Can you work these out from the model? Positions are in its coordinate system, mm. Face numbers are marked on the shaded views. A direction names the side the tool comes from. Give positions to 0.01 mm unless a question says otherwise; leave off trailing zeros. Order: outer loops, then holes, each group sorted by start corner. A loop starts at its lowest first (then second) coordinate and runs counter-clockwise, first axis right, second up. Notation, with made-up numbers: M 82,20.5 L 136,20.5 A22 cw 136,30.5 Z; hole C 16.25,69.25 d8. An arc over 180 degrees is marked long. Answer as a JSON object with one key per item and string values.
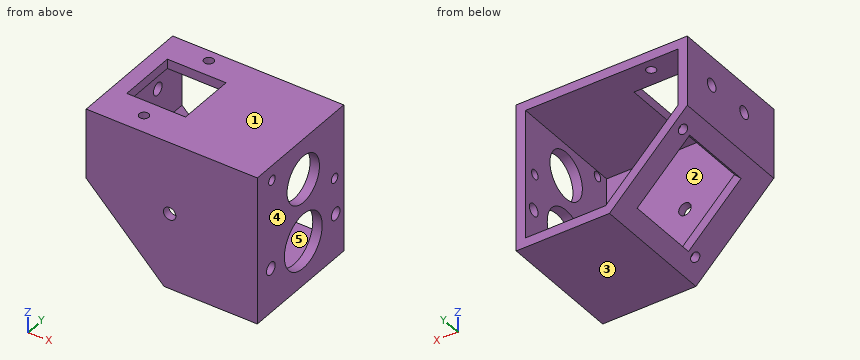
Autodesk Inventor part; units mm, degrees
ref_plane "YZ Plane" through (0, 0, 0) normal (1, 0, 0) x (0, 1, 0)
ref_plane "XZ Plane" through (0, 0, 0) normal (0, 1, 0) x (-1, 0, 0)
ref_plane "XY Plane" through (0, 0, 0) normal (0, 0, 1) x (1, 0, 0)
sketch "Sketch1" plane through (0, 0, 0) normal (0, 1, 0) x (-1, 0, 0)
  line L0 (0, -4) -> (15, -4) construction
  line L1 (15, -4) -> (15, -12) construction
  line L2 (15, -12) -> (-4.6836, -12) construction
  line L3 (0, 0) -> (19.4569, 0)
  line L4 (19.4569, 0) -> (19.4569, -7.2603)
  line L5 (10.2172, -16.5) -> (0, -16.5)
  line L6 (0, -16.5) -> (0, 0)
  line L7 (-1.2, 1.2) -> (20.6569, 1.2)
  line L8 (20.6569, 1.2) -> (20.6569, -7.7574)
  line L9 (10.7142, -17.7) -> (-1.2, -17.7)
  line L10 (-1.2, -17.7) -> (-1.2, 1.2)
  line L11 (10.2172, -16.5) -> (19.4569, -7.2603)
  line L12 (20.6569, -7.7574) -> (10.7142, -17.7)
  line L13 (15, -12) -> (15.7071, -12.7071) construction
  line L14 (17.4749, -6.4749) -> (12.5251, -1.5251) construction
  line L15 (12.5251, -1.5251) -> (13.2676, -0.7827) construction
  line L16 (17.4749, -6.4749) -> (18.2173, -5.7324) construction
  line L17 (18.2173, -5.7324) -> (13.2676, -0.7827) construction
  line L18 (15, -12) -> (16.1863, -13.1863) construction
  point P0 (15, -8)
  dimension "d0" = 1.2
  dimension "d1" = 1.2
  dimension "d2" = 1.2
  dimension "d3" = 4
  dimension "d4" = 4.5
  dimension "d5" = 8
  dimension "d6" = 15
  dimension "d8" = 135
  dimension "d9" = 1.2
  dimension "d10" = 1.2
  dimension "d11" = 1
  dimension "d12" = 7
  dimension "d13" = 45
  dimension "d20" = 7
  dimension "d21" = 1.05
  dimension "d49" = 1.2395
  dimension "d68" = 4.4569
  dimension "d69" = 8
extrude "Extrusion1" add sketch "Sketch1" along normal mid plane 15
sketch "Sketch2" plane through (1.2, -7.5, -17.7) normal (1, 0, 0) x (0, 0, -1)
  circle A0 centre (-5.7, 7.5) radius 3.5
  circle A1 centre (-13.7, 7.5) radius 3
  circle A2 centre (-10.4, 13.3) radius 0.6
  circle A3 centre (-17, 1.7) radius 0.6
  line L0 (-10.4, 13.3) -> (-17, 1.7) construction
  line L1 (-16.7, 7.5) -> (-16.7, 7.5)
  circle A4 centre (-9.7, 1.5) radius 0.8
  line L2 (0, 0) -> (-18.9, 0)
  line L3 (-13.7, 7.5) -> (-5.7, 7.5) construction
  circle A5 centre (-5.7, 13.5) radius 0.8
  circle A6 centre (-5.7, 1.5) radius 0.8
  line L4 (-5.7, 1.5) -> (-5.7, 13.5) construction
  point P0 (-17.7, 7.5)
  point P1 (-5.7, 7.5)
  point P2 (-9.7, 7.5)
  dimension "d22" = 7
  dimension "d23" = 6
  dimension "d56" = 5.8
  dimension "d57" = 3.3
  dimension "d58" = 1.2
  dimension "d59" = 3
  dimension "d66" = 1.6
  dimension "d67" = 1.5
  dimension "d74" = 6
extrude "Extrusion2" cut sketch "Sketch2" against normal blind 3 contours A0 | A1 | A2 | A3 | A5 | A6
sketch "Sketch3" plane through (-20.6569, -7.5, 1.2) normal (-1, 0, 0) x (0, 0, 1)
  circle A0 centre (-3.7, 10.5) radius 0.8
  circle A1 centre (-5.2, 7.5) radius 0.8 construction
  circle A2 centre (-3.7, 4.5) radius 0.8
  line L0 (-11.5, 6.75) -> (-11.5, 8.25)
  line L1 (-9.9, 6.75) -> (-9.9, 8.25)
  arc A3 (-9.9, 8.25) -> (-11.5, 8.25) centre (-10.7, 8.25) ccw
  arc A4 (-11.5, 6.75) -> (-9.9, 6.75) centre (-10.7, 6.75) ccw
  line L2 (-3.7, 4.5) -> (-3.7, 10.5) construction
  point P0 (-1.2, 7.5)
  point P1 (-5.2, 7.5)
  point P2 (-10.7, 7.5)
  point P3 (-11.5, 7.5)
  point P4 (-3.7, 7.5)
  dimension "d28" = 1.6
  dimension "d32" = 5.5
  dimension "d52" = 1.5
  dimension "d53" = 0.8
  dimension "d64" = 6
  dimension "d65" = 1.5
extrude "Extrusion3" cut sketch "Sketch3" against normal blind 2 contours A0 | A2
sketch "Sketch4" plane through (-20.6569, -7.5, -7.7574) normal (-0.7071, 0, -0.7071) x (-0.7071, 0, 0.7071)
  line L0 (-11.75, 12.25) -> (-2.25, 12.25)
  line L1 (-2.25, 12.25) -> (-2.25, 2.75)
  line L2 (-2.25, 2.75) -> (-11.75, 2.75)
  line L3 (-11.75, 2.75) -> (-11.75, 12.25)
  circle A0 centre (-11.75, 13.5) radius 0.6
  circle A1 centre (-2.25, 13.5) radius 0.6
  circle A2 centre (-11.75, 1.5) radius 0.6
  circle A3 centre (-2.25, 1.5) radius 0.6
  point P0 (-9.1213, 7.5)
  point P1 (-7, 7.5)
  point P2 (-7, 7.5)
  point P3 (-7, 7.5)
  point P4 (-11.75, 7.5)
  point P5 (-7, 12.25)
  dimension "d35" = 9.5
  dimension "d36" = 6
  dimension "d37" = 6
  dimension "d38" = 1.2
extrude "Extrusion4" cut sketch "Sketch4" against normal blind 2 contours L0 L1 L2 L3 | A1 | A2
sketch "Sketch5" plane through (-20.6569, 7.5, 1.2) normal (0, 0, 1) x (1, 0, 0)
  line L0 (1.9069, -3.75) -> (9.4069, -3.75)
  line L1 (9.4069, -3.75) -> (9.4069, -11.25)
  line L2 (9.4069, -11.25) -> (1.9069, -11.25)
  line L3 (1.9069, -11.25) -> (1.9069, -3.75)
  circle A0 centre (5.6569, -1.5) radius 0.6
  circle A1 centre (5.6569, -13.5) radius 0.6
  arc A2 (13.6569, -12.7) -> (13.6569, -14.3) centre (13.6569, -13.5) ccw
  arc A3 (17.6569, -14.3) -> (17.6569, -12.7) centre (17.6569, -13.5) ccw
  line L4 (13.6569, -12.7) -> (17.6569, -12.7)
  line L5 (13.6569, -14.3) -> (17.6569, -14.3)
  point P0 (20.6569, -7.5)
  point P1 (5.6569, -7.5)
  point P2 (5.6569, -7.5)
  point P3 (5.6569, -7.5)
  point P4 (9.4069, -7.5)
  point P5 (5.6569, -3.75)
  point P6 (15.6569, -12.7)
  dimension "d41" = 7.5
  dimension "d42" = 6
  dimension "d43" = 6
  dimension "d44" = 1.2
  dimension "d70" = 1.6
  dimension "d71" = 6
  dimension "d72" = 10
  dimension "d73" = 4
extrude "Extrusion5" cut sketch "Sketch5" against normal blind 2 contours L0 L1 L2 L3 | A0 | A1
sketch "Sketch6" plane through (0, -7.5, 0) normal (0, -1, 0) x (1, 0, 0)
  line L0 (1.2, -17.7) -> (1.2, 1.2)
  line L1 (1.2, 1.2) -> (-20.6569, 1.2)
  line L2 (-20.6569, 1.2) -> (-20.6569, -7.7574)
  line L3 (-20.6569, -7.7574) -> (-10.7142, -17.7)
  line L4 (-10.7142, -17.7) -> (1.2, -17.7)
  line L5 (-15, -4) -> (-15, -12) construction
  line L6 (1.2, -10.187) -> (1.2, -11.787)
  circle A0 centre (-15, -8) radius 0.8
  circle A1 centre (-10, -8) radius 0.8
  point P0 (0, 0)
  dimension "d61" = 1.6
  dimension "d62" = 5
extrude "Extrusion6" add sketch "Sketch6" along normal blind 1 contours L4 L3 L2 L1 L0 | A0
properties part number "tactic2 chassis2"
1) I want a section at B-B on y = 1.75. Write out the boundary of the cut face in (x, z).
Results found:
{"outline": "M -20.66,-7.76 L -19.07,-9.35 L -18.22,-8.5 L -19.46,-7.26 L -19.46,0 L -18.75,0 L -18.75,1.2 L -20.66,1.2 Z; M -12.35,-16.07 L -10.71,-17.7 L 1.2,-17.7 L 1.2,-15.03 L 0,-15.03 L 0,-16.5 L -10.22,-16.5 L -11.5,-15.22 Z; M -11.25,0 L 0,0 L 0,-1.56 L 1.2,-1.56 L 1.2,1.2 L -11.25,1.2 Z; M 0,-8.97 L 1.2,-8.97 L 1.2,-6.44 L 0,-6.44 Z"}
2) Thinking about a two-plate mould opening in X: for the marked faces 3, 4 and 5, which applies, pulls with the +X half, pulls with the -X half, needs draft (parallel to the pull), parting line crosses it, or undercut?
Results found:
{"face 3": "needs draft", "face 4": "pulls with the +X half", "face 5": "undercut"}
3) I want a section at A-A on z = -4. Write out the boundary of the cut face in (x, y).
Results found:
{"outline": "M -20.66,-8.5 L 1.2,-8.5 L 1.2,-3 L 0,-3 L 0,-7.5 L -19.46,-7.5 L -19.46,7.5 L -20.66,7.5 Z; M 0,3 L 1.2,3 L 1.2,7.5 L 0,7.5 Z"}
4) I need wall thicknesses on L1, parallel to Y at x = 0.45, z = -12; L2, parallel to Y at x = 0.95, z = -7.3; L3, parallel to Z at x = -1.25, y = 7. Which ranges of each line are inside material? Lowest first, please.
Results found:
{"L1": "y = -8.5 to -6.8, -5.2 to -3.5, 3.5 to 5.2, 6.8 to 7.5", "L2": "y = -8.5 to 5.2, 6.4 to 7.5", "L3": "z = -17.7 to -16.5, 0 to 1.2"}
5) I'm going to push flat-ended pins straight in: pin 1 Ø1.4 at (y, z) = (-6, -12) entering from +X; pin 2 Ø1.4 at (y, z) = (6, -12) entering from -X; pin 3 Ø1 at (x, z) = (-10, -8) entering from +Y; pin 4 Ø0.7 at (x, y) = (-15, 6) entering from +Z. Where does each tip first touch, or does it pass through?
Results found:
{"pin 1": "stops at x = -14.02", "pin 2": "stops at x = -17.11", "pin 3": "passes through", "pin 4": "stops at z = -11.37"}
6) I want a section at D-D on x = -6.5. Write out the boundary of the cut face in (y, z), and give its area (3 significant figures).
Results found:
{"outline": "M -8.5,-17.7 L 7.5,-17.7 L 7.5,-16.5 L -7.5,-16.5 L -7.5,0 L 7.5,0 L 7.5,1.2 L -8.5,1.2 Z", "area": "54.9 mm²"}
7) For the marked faces 1 and 2, which set-ups out of +Z, -Z, +X, -X, +Y, -Y let a thin tool reach every point of the face, with its end or its side?
Results found:
{"face 1": "+Z, +X, -X, +Y, -Y", "face 2": "+Y"}
8) I want a section at C-C on x = -16.75. Write out the boundary of the cut face in (y, z), and give its area (3 significant figures).
Results found:
{"outline": "M -8.5,-11.66 L -4.75,-11.66 L -4.75,-9.97 L -7.5,-9.97 L -7.5,0 L -3.75,0 L -3.75,1.2 L -8.5,1.2 Z; M 3.75,0 L 7.5,0 L 7.5,1.2 L 3.75,1.2 Z; M 4.75,-11.66 L 7.5,-11.66 L 7.5,-9.97 L 4.75,-9.97 Z", "area": "31.2 mm²"}
